Read the model definition and answer for the solid it produces. Units are mm, in the model's axes. A direction names the side the tool comes from. Round coordinates to 2 decimals unless told otherwise and drop trailing zeros. Write each loop counter-clockwise with the first axis right and the second up, starting at its lowest first coordinate (ties: lowest second). Pieces come first, ordered by that corner, then holes.
from build123d import *
from build123d.topology import SkipClean

# Parameters (mm, degrees)
SKETCH1_R           = 38
SKETCH1_R_2         = 3.25
BOSS_EXTRUDE1_DEPTH = 5
BOSS_EXTRUDE2_START = 90
BOSS_EXTRUDE2_DEPTH = 90
BOSS_EXTRUDE3_START = 5
BOSS_EXTRUDE3_DEPTH = 5
CUT_EXTRUDE1_REACH  = 113.477
SKETCH4_R           = 1.5
BOSS_EXTRUDE5_START = -95
BOSS_EXTRUDE5_DEPTH = 120
CUT_EXTRUDE2_REACH  = 135.424
SKETCH7_R           = 1.5
CUT_EXTRUDE3_REACH  = 115.525
BOSS_EXTRUDE6_DEPTH = 25


with BuildPart() as part:
    # Sketch1 → Boss-Extrude1 (new body)
    with BuildSketch(Plane.XY):
        Circle(SKETCH1_R)
        with Locations((-28.5, 0)):
            Circle(SKETCH1_R_2, mode=Mode.SUBTRACT)
        with Locations((28.5, 0)):
            Circle(SKETCH1_R_2, mode=Mode.SUBTRACT)
        with BuildLine():
            Line((-28.5, -6.25), (28.5, -6.25))
            ThreePointArc((28.5, -6.25), (32.067319136, -8.114790357), (32.572245062, -12.108317457))
            ThreePointArc((32.572245062, -12.108317457), (0, -34.75), (-32.572245062, -12.108317457))
            ThreePointArc((-32.572245062, -12.108317457), (-32.067319136, -8.114790357), (-28.5, -6.25))
        make_face(mode=Mode.SUBTRACT)
        with BuildLine():
            Line((-28.5, 6.25), (28.5, 6.25))
            ThreePointArc((28.5, 6.25), (32.067319136, 8.114790357), (32.572245062, 12.108317457))
            ThreePointArc((32.572245062, 12.108317457), (0, 34.75), (-32.572245062, 12.108317457))
            ThreePointArc((-32.572245062, 12.108317457), (-32.067319136, 8.114790357), (-28.5, 6.25))
        make_face(mode=Mode.SUBTRACT)
        with BuildLine():
            Line((23.161460874, 3.25), (-23.161460874, 3.25))
            ThreePointArc((-23.161460874, 3.25), (-22.25, 0), (-23.161460874, -3.25))
            Line((-23.161460874, -3.25), (23.161460874, -3.25))
            ThreePointArc((23.161460874, -3.25), (22.25, 0), (23.161460874, 3.25))
        make_face(mode=Mode.SUBTRACT)
    extrude(amount=BOSS_EXTRUDE1_DEPTH)

    # Sketch2 → Boss-Extrude2 (add)
    with BuildSketch(Plane(origin=(0, 0, 0), x_dir=(-1, 0, 0), z_dir=(0, 0, -1)).offset(BOSS_EXTRUDE2_START)):
        with BuildLine():
            Line((-37.860764652, -3.25), (37.860764652, -3.25))
            ThreePointArc((37.860764652, -3.25), (37.701481777, -4.753763962), (37.482495915, -6.25))
            Line((37.482495915, -6.25), (-37.482495915, -6.25))
            ThreePointArc((-37.482495915, -6.25), (-37.701481777, -4.753763962), (-37.860764652, -3.25))
        make_face()
        with BuildLine():
            Line((-37.482495915, 6.25), (37.482495915, 6.25))
            ThreePointArc((37.482495915, 6.25), (37.701481777, 4.753763962), (37.860764652, 3.25))
            Line((37.860764652, 3.25), (-37.860764652, 3.25))
            ThreePointArc((-37.860764652, 3.25), (-37.701481777, 4.753763962), (-37.482495915, 6.25))
        make_face()
    extrude(amount=-BOSS_EXTRUDE2_DEPTH)

    # Sketch3 → Boss-Extrude3 (add)
    with SkipClean():  # the faces are left unmerged after this step: merging them gives an invalid solid
        with BuildSketch(Plane(origin=(0, 0, -90), x_dir=(-1, 0, 0), z_dir=(0, 0, -1)).offset(BOSS_EXTRUDE3_START)):
            with BuildLine():
                ThreePointArc((37.860764652, 3.25), (37.701481777, 4.753763962), (37.482495915, 6.25))
                ThreePointArc((37.482495915, 6.25), (0, 38), (-37.482495915, 6.25))
                ThreePointArc((-37.482495915, 6.25), (-37.701481777, 4.753763962), (-37.860764652, 3.25))
                ThreePointArc((-37.860764652, 3.25), (-38, 0), (-37.860764652, -3.25))
                ThreePointArc((-37.860764652, -3.25), (-37.701481777, -4.753763962), (-37.482495915, -6.25))
                ThreePointArc((-37.482495915, -6.25), (0, -38), (37.482495915, -6.25))
                ThreePointArc((37.482495915, -6.25), (37.701481777, -4.753763962), (37.860764652, -3.25))
                ThreePointArc((37.860764652, -3.25), (38, 0), (37.860764652, 3.25))
            make_face()
            with BuildLine():
                ThreePointArc((-28.5, 3.25), (-31.75, 0), (-28.5, -3.25))
                ThreePointArc((-28.5, -3.25), (-25.25, 0), (-28.5, 3.25))
            make_face(mode=Mode.SUBTRACT)
            with BuildLine():
                ThreePointArc((28.5, 3.25), (25.25, 0), (28.5, -3.25))
                ThreePointArc((28.5, -3.25), (31.75, 0), (28.5, 3.25))
            make_face(mode=Mode.SUBTRACT)
        extrude(amount=-BOSS_EXTRUDE3_DEPTH)

    # Sketch4 → Cut-Extrude1 (cut, up to next)
    with BuildSketch(Plane(origin=(0, -6.25, 0), x_dir=(1, 0, 0), z_dir=(0, 1, 0)), mode=Mode.PRIVATE) as cut_extrude1_sk1:
        with Locations(Location((-24.5, 62, 0), (0, 0, 180))):
            Circle(SKETCH4_R)
    cut_extrude1_tool1 = extrude(cut_extrude1_sk1.sketch, amount=CUT_EXTRUDE1_REACH, mode=Mode.PRIVATE) & part.part
    # Sketch4 → Cut-Extrude1 (cut, up to next)
    with BuildSketch(Plane(origin=(0, -6.25, 0), x_dir=(1, 0, 0), z_dir=(0, 1, 0)), mode=Mode.PRIVATE) as cut_extrude1_sk2:
        with Locations(Location((24.5, 62, 0), (0, 0, 180))):
            Circle(SKETCH4_R)
    cut_extrude1_tool2 = extrude(cut_extrude1_sk2.sketch, amount=CUT_EXTRUDE1_REACH, mode=Mode.PRIVATE) & part.part
    # Sketch4 → Cut-Extrude1 (cut, up to next)
    with BuildSketch(Plane(origin=(0, -6.25, 0), x_dir=(1, 0, 0), z_dir=(0, 1, 0)), mode=Mode.PRIVATE) as cut_extrude1_sk3:
        with Locations(Location((24.5, 4, 0), (0, 0, 180))):
            Circle(SKETCH4_R)
    cut_extrude1_tool3 = extrude(cut_extrude1_sk3.sketch, amount=CUT_EXTRUDE1_REACH, mode=Mode.PRIVATE) & part.part
    # Sketch4 → Cut-Extrude1 (cut, up to next)
    with BuildSketch(Plane(origin=(0, -6.25, 0), x_dir=(1, 0, 0), z_dir=(0, 1, 0)), mode=Mode.PRIVATE) as cut_extrude1_sk4:
        with Locations(Location((-24.5, 4, 0), (0, 0, 180))):
            Circle(SKETCH4_R)
    cut_extrude1_tool4 = extrude(cut_extrude1_sk4.sketch, amount=CUT_EXTRUDE1_REACH, mode=Mode.PRIVATE) & part.part
    add(cut_extrude1_tool1.solids().sort_by_distance((-24.5, -6.25, -62))[0], mode=Mode.SUBTRACT)
    add(cut_extrude1_tool2.solids().sort_by_distance((24.5, -6.25, -62))[0], mode=Mode.SUBTRACT)
    add(cut_extrude1_tool3.solids().sort_by_distance((24.5, -6.25, -4))[0], mode=Mode.SUBTRACT)
    add(cut_extrude1_tool4.solids().sort_by_distance((-24.5, -6.25, -4))[0], mode=Mode.SUBTRACT)

    # Sketch6 → Boss-Extrude5 (add)
    with SkipClean():  # the faces are left unmerged after this step: merging them gives an invalid solid
        with BuildSketch(Plane(origin=(0, 0, -95), x_dir=(-1, 0, 0), z_dir=(0, 0, -1)).offset(BOSS_EXTRUDE5_START)):
            with BuildLine():
                Line((-34.437443285, 6.25), (34.437443285, 6.25))
                ThreePointArc((34.437443285, 6.25), (34.675570658, 4.754450501), (34.848780466, 3.25))
                Line((34.848780466, 3.25), (-34.848780466, 3.25))
                ThreePointArc((-34.848780466, 3.25), (-34.675570658, 4.754450501), (-34.437443285, 6.25))
            make_face()
        extrude(amount=BOSS_EXTRUDE5_DEPTH)

    # Sketch7 → Cut-Extrude2 (cut, up to next)
    with BuildSketch(Plane(origin=(0, 6.25, 0), x_dir=(1, 0, 0), z_dir=(0, 1, 0)), mode=Mode.PRIVATE) as cut_extrude2_sk1:
        with Locations(Location((-22, 113, 0), (0, 0, 180))):
            Circle(SKETCH7_R)
    cut_extrude2_tool1 = extrude(cut_extrude2_sk1.sketch, amount=-CUT_EXTRUDE2_REACH, mode=Mode.PRIVATE) & part.part
    # Sketch7 → Cut-Extrude2 (cut, up to next)
    with BuildSketch(Plane(origin=(0, 6.25, 0), x_dir=(1, 0, 0), z_dir=(0, 1, 0)), mode=Mode.PRIVATE) as cut_extrude2_sk2:
        with Locations(Location((22, 113, 0), (0, 0, 180))):
            Circle(SKETCH7_R)
    cut_extrude2_tool2 = extrude(cut_extrude2_sk2.sketch, amount=-CUT_EXTRUDE2_REACH, mode=Mode.PRIVATE) & part.part
    # Sketch7 → Cut-Extrude2 (cut, up to next)
    with BuildSketch(Plane(origin=(0, 6.25, 0), x_dir=(1, 0, 0), z_dir=(0, 1, 0)), mode=Mode.PRIVATE) as cut_extrude2_sk3:
        with Locations(Location((22, 25, 0), (0, 0, 180))):
            Circle(SKETCH7_R)
    cut_extrude2_tool3 = extrude(cut_extrude2_sk3.sketch, amount=-CUT_EXTRUDE2_REACH, mode=Mode.PRIVATE) & part.part
    # Sketch7 → Cut-Extrude2 (cut, up to next)
    with BuildSketch(Plane(origin=(0, 6.25, 0), x_dir=(1, 0, 0), z_dir=(0, 1, 0)), mode=Mode.PRIVATE) as cut_extrude2_sk4:
        with Locations(Location((-22, 25, 0), (0, 0, 180))):
            Circle(SKETCH7_R)
    cut_extrude2_tool4 = extrude(cut_extrude2_sk4.sketch, amount=-CUT_EXTRUDE2_REACH, mode=Mode.PRIVATE) & part.part
    add(cut_extrude2_tool1.solids().sort_by_distance((-22, 6.25, -113))[0], mode=Mode.SUBTRACT)
    add(cut_extrude2_tool2.solids().sort_by_distance((22, 6.25, -113))[0], mode=Mode.SUBTRACT)
    add(cut_extrude2_tool3.solids().sort_by_distance((22, 6.25, -25))[0], mode=Mode.SUBTRACT)
    add(cut_extrude2_tool4.solids().sort_by_distance((-22, 6.25, -25))[0], mode=Mode.SUBTRACT)

    # Sketch8 → Cut-Extrude3 (cut, up to next)
    with BuildSketch(Plane(origin=(0, 0, -95), x_dir=(-1, 0, 0), z_dir=(0, 0, -1)), mode=Mode.PRIVATE) as cut_extrude3_sk1:
        with BuildLine():
            Line((-34.437443285, 6.25), (34.437443285, 6.25))
            ThreePointArc((34.437443285, 6.25), (0, 35), (-34.437443285, 6.25))
        make_face()
    cut_extrude3_tool1 = extrude(cut_extrude3_sk1.sketch, amount=-CUT_EXTRUDE3_REACH, mode=Mode.PRIVATE) & part.part
    add(cut_extrude3_tool1.solids().sort_by_distance((0, 18.284736, -95))[0], mode=Mode.SUBTRACT)

    # Sketch9 → Boss-Extrude6 (add)
    with SkipClean():  # the faces are left unmerged after this step: merging them gives an invalid solid
        with BuildSketch(Plane(origin=(0, 0, -95), x_dir=(-1, 0, 0), z_dir=(0, 0, -1))):
            with BuildLine():
                Line((-34.848780466, -3.25), (34.848780466, -3.25))
                ThreePointArc((34.848780466, -3.25), (34.675570658, -4.754450501), (34.437443285, -6.25))
                Line((34.437443285, -6.25), (-34.437443285, -6.25))
                ThreePointArc((-34.437443285, -6.25), (-34.675570658, -4.754450501), (-34.848780466, -3.25))
            make_face()
        extrude(amount=BOSS_EXTRUDE6_DEPTH)


solid = part.part
Q1. Section A-A (x = 0) is taken. Determine the outline of the cut face in (y, z), then the cut area to 3 significant figures.
Verdict:
outline: (-38, -95) - (-6.25, -95) - (-6.25, -120) - (-3.25, -120) - (-3.25, -95) - (3.25, -95) - (3.25, -120) - (6.25, -120) - (6.25, 5) - (3.25, 5) - (3.25, -90) - (-3.25, -90) - (-3.25, 5) - (-6.25, 5) - (-6.25, -90) - (-38, -90) - close; (-38, 0) - (-34.75, 0) - (-34.75, 5) - (-38, 5) - close; (34.75, 0) - (38, 0) - (38, 5) - (34.75, 5) - close; (35, -95) - (38, -95) - (38, -90) - (35, -90) - close
area: 989 mm2
Q2. Section D-D (z = -62) is taken. Determine the outline of the cut face in (x, y).
Verdict:
outline: (-37.86, -3.25) arc R38 ccw to (-37.48, -6.25) - (-26, -6.25) - (-26, -3.25) - close; (-37.86, 3.25) - (37.86, 3.25) arc R38 ccw to (37.48, 6.25) - (-37.48, 6.25) arc R38 ccw to start; (-23, -6.25) - (23, -6.25) - (23, -3.25) - (-23, -3.25) - close; (26, -6.25) - (37.48, -6.25) arc R38 ccw to (37.86, -3.25) - (26, -3.25) - close
Q3. Straight lines are drawn through the part: probe 1 along X at (y, z) = (0, 2); probe 2 along Z at (x, y) = (24.5, -4.2); probe 3 along X at (y, z) = (0, -91). For each, find the intervals that lie inside material, in ascending order.
Verdict:
probe 1: x = -38 to -31.75, -25.25 to -22.25, 22.25 to 25.25, 31.75 to 38
probe 2: z = -120 to -63.5, -60.5 to -5.5, -2.5 to 5
probe 3: x = -38 to -31.75, -25.25 to 25.25, 31.75 to 38
Q4. Flat-ended cylindrical pins translate along their axes: pin 1 Ø3.5 at (x, z) = (-24.5, -4) entering from +Y; pin 2 Ø1.8 at (x, z) = (22, -25) entering from +Y; pin 3 Ø4 at (x, z) = (-22, -25) entering from -Y. Find the tip coordinate at first contact, or state that the pin passes through.
Verdict:
pin 1: stops at y = 6.25
pin 2: stops at y = -3.25
pin 3: stops at y = -6.25
Q5. Which of the six approach directions +Z, -Z, +X, -X, +Y, -Y give full straight-line access (tool end or side, diameter ignored) to faces 4 (the cylindrical face through (22.195, 4.771, -111.513)), 5 (the flat face through (-34, 0, -90)), 6 (the flat face through (0, 0, -95))?
Verdict:
face 4: +Y
face 5: +X, -X
face 6: -Z, +X, -X
Q6. Determine the mould class of faces 1 (the cylindrical face through (34.68, 4.73, -107.32)), 2 (the flat face through (25, 0, 0)), 3 (the flat face through (3, 35.1, -90)) for opening direction Y: pulls with the +Y half, pulls with the -Y half, needs draft (parallel to the pull), parting line crosses it, or undercut.
Verdict:
face 1: pulls with the +Y half
face 2: undercut
face 3: needs draft
Q7. Section C-C (y = 0) is taken. Determine the outline of the cut face in (x, z), then the cut area to 4 significant figures.
Verdict:
outline: (-38, -95) - (-31.75, -95) - (-31.75, -90) - (-38, -90) - close; (-38, 0) - (-31.75, 0) - (-31.75, 5) - (-38, 5) - close; (-25.25, -95) - (25.25, -95) - (25.25, -90) - (-25.25, -90) - close; (-25.25, 0) - (-22.25, 0) - (-22.25, 5) - (-25.25, 5) - close; (22.25, 0) - (25.25, 0) - (25.25, 5) - (22.25, 5) - close; (31.75, -95) - (38, -95) - (38, -90) - (31.75, -90) - close; (31.75, 0) - (38, 0) - (38, 5) - (31.75, 5) - close
area: 407.5 mm2
Q8. Section B-B (z = -43) is taken. Determine the outline of the cut face in (x, y), then the cut area to 3 significant figures.
Verdict:
outline: (-37.86, -3.25) arc R38 ccw to (-37.48, -6.25) - (37.48, -6.25) arc R38 ccw to (37.86, -3.25) - close; (-37.86, 3.25) - (37.86, 3.25) arc R38 ccw to (37.48, 6.25) - (-37.48, 6.25) arc R38 ccw to start
area: 452 mm2
